Check sheet for the drawn part. Datum: minimum x, y, z corner. Units: mm. A direction names the side the tool comes from. Give positions to 0.01 mm unless a question says otherwise; leave off trailing zeros. Write each loop counter-clockwise with the first axis right and the second up, starting at its lowest first coordinate (ties: lowest second). Pieces come first, ordered by that corner, then holes.
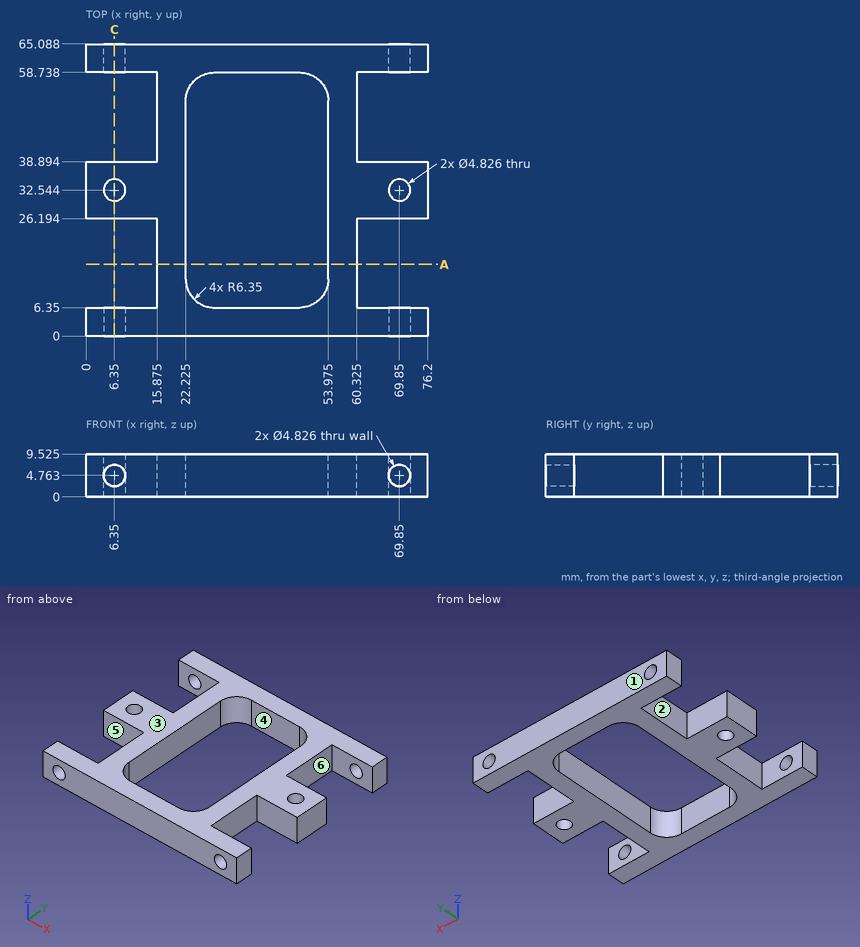
1) Gauge pin test, flat ends, axial feed: pin 1 (5 mm diameter, centred on x = 54, y = 42.5, fed in from -Z); pin 2 (3 mm diameter, centred on x = 6.35, y = 32.54, fed in from -Z); pin 3 (5 mm diameter, centred on y = 51, z = 6.5, fed in from +X) (1 decimal); pin 4 (5 mm diameter, centred on y = 49.5, z = 3.5, fed in from -X) (1 decimal). Record the tip position at first contact, or that the pin passes through.
2) Sectioned sample at C-C on x = 6.35. Give the number of separate pieces and of enclosed holes in the cut face, then the cut area to 3 significant figures.
3) Scan lines: L1, parallel to X at y = 5.5, z = 4.5; L2, parallel to Y at x = 72.5, z = 4.5; L3, parallel to Y at x = 32, z = 3. Record each from-to range of solid material in increasing order.
4) Draft check along Y on the marked faces 1, 2 and 3. Enter one of: +Y half, -Y half, draft (parallel to the pull), parting line (faces both ways), or undercut.
5) Access from +Z, -Z, +X, -X, +Y, -Y to the whole of each face (thin tool, end or side, straight path). Record for the marked faces 4, 5 and 6.
6) Sectioned sample at A-A on y = 16. Record the boundary of the cut face in (x, z) (1 decimal).
Answers below:
1. pin 1: stops at z = 0
1. pin 2: passes through
1. pin 3: stops at x = 60.3
1. pin 4: stops at x = 15.9
2. separate pieces: 6
2. enclosed holes: 0
2. area: 135 mm2
3. L1: x = 0 to 3.95, 8.75 to 67.45, 72.25 to 76.2
3. L2: y = 0 to 6.35, 26.19 to 38.89, 58.74 to 65.09
3. L3: y = 0 to 6.35, 58.74 to 65.09
4. face 1: +Y half
4. face 2: undercut
4. face 3: draft
5. face 4: +Z, -Z
5. face 5: +Z, -Z, -X
5. face 6: +Z, -Z, +X
6. outline: (15.9, 0) - (22.2, 0) - (22.2, 9.5) - (15.9, 9.5) - close; (54, 0) - (60.3, 0) - (60.3, 9.5) - (54, 9.5) - close
